CAD build for the part. Positions are in the model's coordinates, mm. A direction names the side the tool comes from. Coordinates: 2 decimals unless noted, no trailing zeros. Loops run counter-clockwise (first coordinate to the right, second up) from the corner with the lowest first, then second, coordinate; pieces in that order, holes last. Notation, with made-up numbers: M 65.5,-4 L 98.5,-4 A17 ccw 98.5,20 Z; hole C 8,86.25 d4. An arc over 180 degrees is marked long. Answer as a JSON object with one key per item and string values. Group by question number.
```python
from build123d import *

# Parameters (mm, degrees)
F1_DEPTH  = 1
F2_DEPTH  = 2
F3_DEPTH  = 3
F4_DEPTH  = 4
F5_DEPTH  = 5
F6_DEPTH  = 6
F7_DEPTH  = 7
F8_DEPTH  = 8
F9_DEPTH  = 9
F10_DEPTH = 10
F11_DEPTH = 11
F12_DEPTH = 12
F13_DEPTH = 13
F14_DEPTH = 14
F15_DEPTH = 25


with BuildPart() as f1:
    # F0 (on Front) → F1 (new body)
    with BuildSketch(Plane.XZ):
        Polygon((-0.013426, -0.007751), (0.013426, -0.007751), (0, 0.015503), align=None)
    extrude(amount=F1_DEPTH)

    # F0 (on Front) → F2 (join)
    with BuildSketch(Plane.XZ):
        Polygon((0, 0.015503), (-0.026852, 0.015503), (-0.013426, -0.007751), align=None)
    extrude(amount=F2_DEPTH)

    # F0 (on Front) → F3 (join)
    with BuildSketch(Plane.XZ):
        Polygon((0.026852, 0.015503), (0, 0.062012), (-0.026852, 0.015503), (0, 0.015503), align=None)
    extrude(amount=F3_DEPTH)

    # F0 (on Front) → F4 (join)
    with BuildSketch(Plane.XZ):
        Polygon((0.053704, -0.031006), (0.107407, 0.062012), (0, 0.062012), (0.026852, 0.015503), align=None)
    extrude(amount=F4_DEPTH)

    # F0 (on Front) → F5 (join)
    with BuildSketch(Plane.XZ):
        Polygon((0, -0.124023), (0.214815, -0.124023), (0.107407, 0.062012), (0.053704, -0.031006), align=None)
    extrude(amount=F5_DEPTH)

    # F0 (on Front) → F6 (join)
    with BuildSketch(Plane.XZ):
        Polygon((-0.214815, -0.124023), (0, -0.496094), (0.214815, -0.124023), (0, -0.124023), align=None)
    extrude(amount=F6_DEPTH)

    # F0 (on Front) → F7 (join)
    with BuildSketch(Plane.XZ):
        Polygon((-0.42963, 0.248047), (-0.85926, -0.496094), (0, -0.496094), (-0.214815, -0.124023), align=None)
    extrude(amount=F7_DEPTH)

    # F0 (on Front) → F8 (join)
    with BuildSketch(Plane.XZ):
        Polygon((0, 0.992187), (-1.718519, 0.992187), (-0.85926, -0.496094), (-0.42963, 0.248047), align=None)
    extrude(amount=F8_DEPTH)

    # F0 (on Front) → F9 (join)
    with BuildSketch(Plane.XZ):
        Polygon((1.718519, 0.992188), (0, 3.96875), (-1.718519, 0.992187), (0, 0.992187), align=None)
    extrude(amount=F9_DEPTH)

    # F0 (on Front) → F10 (join)
    with BuildSketch(Plane.XZ):
        Polygon((3.437038, -1.984375), (6.874077, 3.96875), (0, 3.96875), (1.718519, 0.992188), align=None)
    extrude(amount=F10_DEPTH)

    # F0 (on Front) → F11 (join)
    with BuildSketch(Plane.XZ):
        Polygon((0, -7.9375), (13.748153, -7.9375), (6.874077, 3.96875), (3.437038, -1.984375), align=None)
    extrude(amount=F11_DEPTH)

    # F0 (on Front) → F12 (join)
    with BuildSketch(Plane.XZ):
        Polygon((-13.748153, -7.9375), (0, -31.75), (13.748153, -7.9375), (0, -7.9375), align=None)
    extrude(amount=F12_DEPTH)

    # F0 (on Front) → F13 (join)
    with BuildSketch(Plane.XZ):
        Polygon((-27.496307, 15.875), (-54.992613, -31.75), (0, -31.75), (-13.748153, -7.9375), align=None)
    extrude(amount=F13_DEPTH)

    # F0 (on Front) → F14 (join)
    with BuildSketch(Plane.XZ):
        Polygon((0, 63.5), (-109.985226, 63.5), (-54.992613, -31.75), (-27.496307, 15.875), align=None)
    extrude(amount=F14_DEPTH)

    # F0 (on Front) → F15 (join)
    with BuildSketch(Plane.XZ):
        Polygon((109.985226, 63.5), (0, 254), (-109.985226, 63.5), (0, 63.5), align=None)
    extrude(amount=F15_DEPTH)


solid = f1.part
```
Item 1: Pull direction X, two halves, no side cores. Call faces 5 (the flat face through (-54.223, -12.325, 160.083)), 6 (the flat face through (3, -10, 2)), 7 (the flat face through (6.78, -5.92, -20.01)): released by +X, released by -X, zero draft, split by the parting line, or undercut.
Item 2: Drill centre lines: L1, parallel to Z at x = -25, y = -7.25; L2, parallel to Z at x = -22.5, y = -6.25; L3, parallel to Z at x = -41, y = -8.5. Where is each one in solid material? Low to high. Write a range as from..to.
Item 3: Pin check, flat tips, straight feed: pin 1 (12 mm diameter, centred on y = -20.5, z = 26.5, fed in from -X); pin 2 (4 mm diameter, centred on y = -6.5, z = 30.5, fed in from +X); pin 3 (0.6 mm diameter, centred on x = -0.5, z = 0, fed in from -Y); pin 4 (2 mm diameter, centred on x = 4, y = -6, fed in from +Z). Stop position of each tip, or through.
Item 4: Slice it at B-B, the plane x = -45. Write the cut outline in (y, z), then the cut area to 3 significant figures.
Item 5: Slice it at A-A, the plane x = -20. Write the cut outline in (y, z), then the cut area to 3 significant figures.
Item 6: Slice it at D-D, the plane z = 133. Write the cut outline in (x, y).
Item 7: Tool access for faces 1 (the flat face through (-6, -6, -7.938)), 2 (the flat face through (10.36, -5.42, -2.07)), 3 (the flat face through (-28, -13, -13)), 4 (the flat face through (7, -11, -3)): list every direction of +Z, -Z, +X, -X, +Y, -Y with a clear straight run to the whole face (end or side of a thin tool).
Item 8: Slice it at C-C, the plane y = -17.75. Write the cut outline in (x, z), then the cut area to 3 significant figures.
Computed:
{
 "1": {"face 5": "released by -X", "face 6": "undercut", "face 7": "released by +X"},
 "2": {"L1": "-31.75..11.55, 20.2..210.7", "L2": "-31.75..7.22, 24.53..215.03", "L3": "-31.75..182.99"},
 "3": {"pin 1": "through", "pin 2": "x = -17.9", "pin 3": "y = -8", "pin 4": "z = 248.8"},
 "4": {"outline": "M -25,63.5 L -14,63.5 L -14,-14.44 L -13,-14.44 L -13,-31.75 L 0,-31.75 L 0,176.06 L -25,176.06 Z", "area": "4,130 mm2"},
 "5": {"outline": "M -25,63.5 L -14,63.5 L -14,28.86 L 0,28.86 L 0,219.36 L -25,219.36 Z; M -13,-31.75 L 0,-31.75 L 0,2.89 L -13,2.89 Z", "area": "4,830 mm2"},
 "6": {"outline": "M -69.86,-25 L 69.86,-25 L 69.86,0 L -69.86,0 Z"},
 "7": {"face 1": "-Y", "face 2": "+X, +Y, -Y", "face 3": "-Z, +X, -Y", "face 4": "+X, -Y"},
 "8": {"outline": "M -109.99,63.5 L 109.99,63.5 L 0,254 Z", "area": "21,000 mm2"}
}
